```python
from build123d import *

# Parameters (mm, degrees)
SKETCH1_W               = 50.8
SKETCH1_H               = 25.4
SKETCH1_W_2             = 44.45
SKETCH1_H_2             = 19.05
BOSS_EXTRUDE1_DEPTH     = 774.7
SKETCH3_R               = 14.2875
CUT_EXTRUDE2_DEPTH      = 777.578000348
SKETCH2_R               = 6.35
CUT_EXTRUDE1_DEPTH      = 777.578000348
SKETCH4_R               = 2.54
CUT_EXTRUDE3_DEPTH      = 777.578000348
SKETCH5_R               = 2.54
CUT_EXTRUDE4_DEPTH      = 777.578000348
CUT_EXTRUDE5_DEPTH      = 777.578000348
CUT_EXTRUDE5_DEPTH_BACK = 777.578000348
SKETCH6_R               = 3.175
SKETCH8_R               = 2.5796875
CUT_EXTRUDE8_DEPTH      = 777.578000348
SKETCH10_R              = 3.175
SKETCH10_R_2            = 3.3734375
CUT_EXTRUDE9_DEPTH      = 777.578000348
CUT_EXTRUDE10_REACH     = 778.682
SKETCH11_R              = 2.4638
CUT_EXTRUDE11_REACH     = 778.682
SKETCH12_R              = 2.4638
CUT_EXTRUDE12_REACH     = 778.682
SKETCH13_R              = 2.4638


with BuildPart() as part:
    # Sketch1 → Boss-Extrude1 (new body)
    with BuildSketch(Plane(origin=(0, 0, 0), x_dir=(1, 0, 0), z_dir=(0, 1, 0))):
        with Locations((22.225, 9.525)):
            Rectangle(SKETCH1_W, SKETCH1_H)
        with Locations((22.225, 9.525)):
            Rectangle(SKETCH1_W_2, SKETCH1_H_2, mode=Mode.SUBTRACT)
    extrude(amount=BOSS_EXTRUDE1_DEPTH)

    # Sketch3 → Cut-Extrude2 (cut, through all)
    with BuildSketch(Plane.XY.offset(3.175)):
        with Locations((22.225, 81.28)):
            Circle(SKETCH3_R)
    extrude(amount=-CUT_EXTRUDE2_DEPTH, mode=Mode.SUBTRACT)

    # Sketch2 → Cut-Extrude1 (cut, through all)
    with BuildSketch(Plane.XY.offset(3.175)):
        with Locations((22.225, 633.476)):
            Circle(SKETCH2_R)
    extrude(amount=-CUT_EXTRUDE1_DEPTH, mode=Mode.SUBTRACT)

    # Sketch4 → Cut-Extrude3 (cut, through all)
    with BuildSketch(Plane.XY.offset(3.175)):
        with Locations((40.511702836, 42.589037005)):
            Circle(SKETCH4_R)
        with Locations((40.511702836, 119.970962995)):
            Circle(SKETCH4_R)
    extrude(amount=-CUT_EXTRUDE3_DEPTH, mode=Mode.SUBTRACT)

    # Sketch5 → Cut-Extrude4 (cut, through all)
    with BuildSketch(Plane(origin=(0, 0, -22.225), x_dir=(-1, 0, 0), z_dir=(0, 0, -1))):
        with Locations((-10.31875, 612.853770072)):
            Circle(SKETCH5_R)
        with Locations((-34.13125, 612.853770072)):
            Circle(SKETCH5_R)
        with Locations((-10.31875, 654.098229928)):
            Circle(SKETCH5_R)
        with Locations((-34.13125, 654.098229928)):
            Circle(SKETCH5_R)
    extrude(amount=-CUT_EXTRUDE4_DEPTH, mode=Mode.SUBTRACT)

    # Sketch6 → Cut-Extrude5 (cut, two sides: drawn at the far end of the back side and taken through both)
    with BuildSketch(Plane.XY.offset(3.175).offset(-CUT_EXTRUDE5_DEPTH_BACK)):
        with Locations((4.445, 227.076)):
            Circle(SKETCH6_R)
        with Locations((4.445, 328.676)):
            Circle(SKETCH6_R)
    extrude(amount=CUT_EXTRUDE5_DEPTH + CUT_EXTRUDE5_DEPTH_BACK, mode=Mode.SUBTRACT)

    # Sketch8 → Cut-Extrude8 (cut, through all)
    with BuildSketch(Plane.XY.offset(3.175)):
        with Locations((4.445, 315.976)):
            Circle(SKETCH8_R)
        with Locations((4.445, 308.356)):
            Circle(SKETCH8_R)
    extrude(amount=-CUT_EXTRUDE8_DEPTH, mode=Mode.SUBTRACT)

    # Sketch10 → Cut-Extrude9 (cut, through all)
    with BuildSketch(Plane.XY.offset(3.175)):
        with Locations((34.925, 195.58)):
            Circle(SKETCH10_R)
        with Locations((34.925, 391.16)):
            Circle(SKETCH10_R)
        with Locations((34.925, 533.4)):
            Circle(SKETCH10_R)
        with Locations((34.925, 728.98)):
            Circle(SKETCH10_R)
        with Locations((4.445, 728.98)):
            Circle(SKETCH10_R_2)
    extrude(amount=-CUT_EXTRUDE9_DEPTH, mode=Mode.SUBTRACT)

    # Sketch11 → Cut-Extrude10 (cut, up to next)
    with BuildSketch(Plane.ZY.offset(3.175), mode=Mode.PRIVATE) as cut_extrude10_sk1:
        with Locations((-9.525, 762)):
            Circle(SKETCH11_R)
    cut_extrude10_tool1 = extrude(cut_extrude10_sk1.sketch, amount=-CUT_EXTRUDE10_REACH, mode=Mode.PRIVATE) & part.part
    # Sketch11 → Cut-Extrude10 (cut, up to next)
    with BuildSketch(Plane.ZY.offset(3.175), mode=Mode.PRIVATE) as cut_extrude10_sk2:
        with Locations((-9.525, 723.9)):
            Circle(SKETCH11_R)
    cut_extrude10_tool2 = extrude(cut_extrude10_sk2.sketch, amount=-CUT_EXTRUDE10_REACH, mode=Mode.PRIVATE) & part.part
    # Sketch11 → Cut-Extrude10 (cut, up to next)
    with BuildSketch(Plane.ZY.offset(3.175), mode=Mode.PRIVATE) as cut_extrude10_sk3:
        with Locations((-9.525, 558.8)):
            Circle(SKETCH11_R)
    cut_extrude10_tool3 = extrude(cut_extrude10_sk3.sketch, amount=-CUT_EXTRUDE10_REACH, mode=Mode.PRIVATE) & part.part
    # Sketch11 → Cut-Extrude10 (cut, up to next)
    with BuildSketch(Plane.ZY.offset(3.175), mode=Mode.PRIVATE) as cut_extrude10_sk4:
        with Locations((-9.525, 533.4)):
            Circle(SKETCH11_R)
    cut_extrude10_tool4 = extrude(cut_extrude10_sk4.sketch, amount=-CUT_EXTRUDE10_REACH, mode=Mode.PRIVATE) & part.part
    # Sketch11 → Cut-Extrude10 (cut, up to next)
    with BuildSketch(Plane.ZY.offset(3.175), mode=Mode.PRIVATE) as cut_extrude10_sk5:
        with Locations((-9.525, 495.3)):
            Circle(SKETCH11_R)
    cut_extrude10_tool5 = extrude(cut_extrude10_sk5.sketch, amount=-CUT_EXTRUDE10_REACH, mode=Mode.PRIVATE) & part.part
    # Sketch11 → Cut-Extrude10 (cut, up to next)
    with BuildSketch(Plane.ZY.offset(3.175), mode=Mode.PRIVATE) as cut_extrude10_sk6:
        with Locations((-9.525, 50.8)):
            Circle(SKETCH11_R)
    cut_extrude10_tool6 = extrude(cut_extrude10_sk6.sketch, amount=-CUT_EXTRUDE10_REACH, mode=Mode.PRIVATE) & part.part
    # Sketch11 → Cut-Extrude10 (cut, up to next)
    with BuildSketch(Plane.ZY.offset(3.175), mode=Mode.PRIVATE) as cut_extrude10_sk7:
        with Locations((-9.525, 12.7)):
            Circle(SKETCH11_R)
    cut_extrude10_tool7 = extrude(cut_extrude10_sk7.sketch, amount=-CUT_EXTRUDE10_REACH, mode=Mode.PRIVATE) & part.part
    add(cut_extrude10_tool1.solids().sort_by_distance((-3.175, 762, -9.525))[0], mode=Mode.SUBTRACT)
    add(cut_extrude10_tool2.solids().sort_by_distance((-3.175, 723.9, -9.525))[0], mode=Mode.SUBTRACT)
    add(cut_extrude10_tool3.solids().sort_by_distance((-3.175, 558.8, -9.525))[0], mode=Mode.SUBTRACT)
    add(cut_extrude10_tool4.solids().sort_by_distance((-3.175, 533.4, -9.525))[0], mode=Mode.SUBTRACT)
    add(cut_extrude10_tool5.solids().sort_by_distance((-3.175, 495.3, -9.525))[0], mode=Mode.SUBTRACT)
    add(cut_extrude10_tool6.solids().sort_by_distance((-3.175, 50.8, -9.525))[0], mode=Mode.SUBTRACT)
    add(cut_extrude10_tool7.solids().sort_by_distance((-3.175, 12.7, -9.525))[0], mode=Mode.SUBTRACT)

    # Sketch12 → Cut-Extrude11 (cut, up to next)
    with BuildSketch(Plane(origin=(47.625, 0, 0), x_dir=(0, 0, -1), z_dir=(1, 0, 0)), mode=Mode.PRIVATE) as cut_extrude11_sk1:
        with Locations(Location((9.525, 50.8, 0), (0, 0, 180))):
            Circle(SKETCH12_R)
    cut_extrude11_tool1 = extrude(cut_extrude11_sk1.sketch, amount=-CUT_EXTRUDE11_REACH, mode=Mode.PRIVATE) & part.part
    # Sketch12 → Cut-Extrude11 (cut, up to next)
    with BuildSketch(Plane(origin=(47.625, 0, 0), x_dir=(0, 0, -1), z_dir=(1, 0, 0)), mode=Mode.PRIVATE) as cut_extrude11_sk2:
        with Locations((9.525, 114.3)):
            Circle(SKETCH12_R)
    cut_extrude11_tool2 = extrude(cut_extrude11_sk2.sketch, amount=-CUT_EXTRUDE11_REACH, mode=Mode.PRIVATE) & part.part
    # Sketch12 → Cut-Extrude11 (cut, up to next)
    with BuildSketch(Plane(origin=(47.625, 0, 0), x_dir=(0, 0, -1), z_dir=(1, 0, 0)), mode=Mode.PRIVATE) as cut_extrude11_sk3:
        with Locations((9.525, 177.8)):
            Circle(SKETCH12_R)
    cut_extrude11_tool3 = extrude(cut_extrude11_sk3.sketch, amount=-CUT_EXTRUDE11_REACH, mode=Mode.PRIVATE) & part.part
    # Sketch12 → Cut-Extrude11 (cut, up to next)
    with BuildSketch(Plane(origin=(47.625, 0, 0), x_dir=(0, 0, -1), z_dir=(1, 0, 0)), mode=Mode.PRIVATE) as cut_extrude11_sk4:
        with Locations((9.525, 241.3)):
            Circle(SKETCH12_R)
    cut_extrude11_tool4 = extrude(cut_extrude11_sk4.sketch, amount=-CUT_EXTRUDE11_REACH, mode=Mode.PRIVATE) & part.part
    # Sketch12 → Cut-Extrude11 (cut, up to next)
    with BuildSketch(Plane(origin=(47.625, 0, 0), x_dir=(0, 0, -1), z_dir=(1, 0, 0)), mode=Mode.PRIVATE) as cut_extrude11_sk5:
        with Locations((9.525, 304.8)):
            Circle(SKETCH12_R)
    cut_extrude11_tool5 = extrude(cut_extrude11_sk5.sketch, amount=-CUT_EXTRUDE11_REACH, mode=Mode.PRIVATE) & part.part
    # Sketch12 → Cut-Extrude11 (cut, up to next)
    with BuildSketch(Plane(origin=(47.625, 0, 0), x_dir=(0, 0, -1), z_dir=(1, 0, 0)), mode=Mode.PRIVATE) as cut_extrude11_sk6:
        with Locations((9.525, 368.3)):
            Circle(SKETCH12_R)
    cut_extrude11_tool6 = extrude(cut_extrude11_sk6.sketch, amount=-CUT_EXTRUDE11_REACH, mode=Mode.PRIVATE) & part.part
    # Sketch12 → Cut-Extrude11 (cut, up to next)
    with BuildSketch(Plane(origin=(47.625, 0, 0), x_dir=(0, 0, -1), z_dir=(1, 0, 0)), mode=Mode.PRIVATE) as cut_extrude11_sk7:
        with Locations((9.525, 431.8)):
            Circle(SKETCH12_R)
    cut_extrude11_tool7 = extrude(cut_extrude11_sk7.sketch, amount=-CUT_EXTRUDE11_REACH, mode=Mode.PRIVATE) & part.part
    # Sketch12 → Cut-Extrude11 (cut, up to next)
    with BuildSketch(Plane(origin=(47.625, 0, 0), x_dir=(0, 0, -1), z_dir=(1, 0, 0)), mode=Mode.PRIVATE) as cut_extrude11_sk8:
        with Locations(Location((9.525, 495.3, 0), (0, 0, 180))):
            Circle(SKETCH12_R)
    cut_extrude11_tool8 = extrude(cut_extrude11_sk8.sketch, amount=-CUT_EXTRUDE11_REACH, mode=Mode.PRIVATE) & part.part
    # Sketch12 → Cut-Extrude11 (cut, up to next)
    with BuildSketch(Plane(origin=(47.625, 0, 0), x_dir=(0, 0, -1), z_dir=(1, 0, 0)), mode=Mode.PRIVATE) as cut_extrude11_sk9:
        with Locations(Location((9.525, 558.8, 0), (0, 0, 180))):
            Circle(SKETCH12_R)
    cut_extrude11_tool9 = extrude(cut_extrude11_sk9.sketch, amount=-CUT_EXTRUDE11_REACH, mode=Mode.PRIVATE) & part.part
    add(cut_extrude11_tool1.solids().sort_by_distance((47.625, 50.8, -9.525))[0], mode=Mode.SUBTRACT)
    add(cut_extrude11_tool2.solids().sort_by_distance((47.625, 114.3, -9.525))[0], mode=Mode.SUBTRACT)
    add(cut_extrude11_tool3.solids().sort_by_distance((47.625, 177.8, -9.525))[0], mode=Mode.SUBTRACT)
    add(cut_extrude11_tool4.solids().sort_by_distance((47.625, 241.3, -9.525))[0], mode=Mode.SUBTRACT)
    add(cut_extrude11_tool5.solids().sort_by_distance((47.625, 304.8, -9.525))[0], mode=Mode.SUBTRACT)
    add(cut_extrude11_tool6.solids().sort_by_distance((47.625, 368.3, -9.525))[0], mode=Mode.SUBTRACT)
    add(cut_extrude11_tool7.solids().sort_by_distance((47.625, 431.8, -9.525))[0], mode=Mode.SUBTRACT)
    add(cut_extrude11_tool8.solids().sort_by_distance((47.625, 495.3, -9.525))[0], mode=Mode.SUBTRACT)
    add(cut_extrude11_tool9.solids().sort_by_distance((47.625, 558.8, -9.525))[0], mode=Mode.SUBTRACT)

    # Sketch13 → Cut-Extrude12 (cut, up to next)
    with BuildSketch(Plane(origin=(47.625, 0, 0), x_dir=(0, 0, -1), z_dir=(1, 0, 0)), mode=Mode.PRIVATE) as cut_extrude12_sk1:
        with Locations(Location((9.525, 762, 0), (0, 0, 180))):
            Circle(SKETCH13_R)
    cut_extrude12_tool1 = extrude(cut_extrude12_sk1.sketch, amount=-CUT_EXTRUDE12_REACH, mode=Mode.PRIVATE) & part.part
    # Sketch13 → Cut-Extrude12 (cut, up to next)
    with BuildSketch(Plane(origin=(47.625, 0, 0), x_dir=(0, 0, -1), z_dir=(1, 0, 0)), mode=Mode.PRIVATE) as cut_extrude12_sk2:
        with Locations(Location((9.525, 723.9, 0), (0, 0, 180))):
            Circle(SKETCH13_R)
    cut_extrude12_tool2 = extrude(cut_extrude12_sk2.sketch, amount=-CUT_EXTRUDE12_REACH, mode=Mode.PRIVATE) & part.part
    add(cut_extrude12_tool1.solids().sort_by_distance((47.625, 762, -9.525))[0], mode=Mode.SUBTRACT)
    add(cut_extrude12_tool2.solids().sort_by_distance((47.625, 723.9, -9.525))[0], mode=Mode.SUBTRACT)


solid = part.part
```
CAD build for the part. Positions are in the model's coordinates, mm. A direction names the side the tool comes from. Round coordinates to 2 decimals unless told otherwise and drop trailing zeros. Write each loop counter-clockwise with the first axis right and the second up, starting at its lowest first coordinate (ties: lowest second). Pieces come first, ordered by that corner, then holes. Notation, with made-up numbers: (41.25, 34.5) - (96.25, 34.5) arc R21 cw to (96.25, 64.5) - close; hole circle Ø4 at (27.25, 35.25). An arc over 180 degrees is marked (long way). Return JSON: item names as keys, results as strings. Group by question number.
Item 1: 3-axis set-ups, long thin cutter, end or side, ignore diameter. For faces 4 (the face through (-3.175, 382, -9)), 5 (the face through (22, 382, -19.05)): which of +Z, -Z, +X, -X, +Y, -Y reach the whole face in a straight line?
Item 2: Band-saw the part on B-B on y = 475.5. List the corners of the cut face in (x, z) (3 decimals).
Item 3: Probe probe 1 along Z at (x, y) = (26, 384) (3 decimals); probe 2 along Z at (x, y) = (-2, 762) (3 decimals); probe 3 along X at (y, z) = (150.5, -17.5) (3 decimals). List the from-to ranges inside material, lowest first.
Item 4: Mould opens along Y. For faces 1 (the face through (0, 382, -9)), 2 (the face through (25.64, 638.83, 1.61)), 3 (the face through (22, 0, -20)) say: +Y half, -Y half, draft (parallel to the pull), parting line (faces both ways), or undercut.
Resolved:
{
 "1": {"face 4": "+Z, -Z, -X, +Y, -Y", "face 5": "+Y, -Y"},
 "2": {"outline": "(-3.175, -22.225) - (47.625, -22.225) - (47.625, 3.175) - (-3.175, 3.175) - close; hole (0, -19.05) - (44.45, -19.05) - (44.45, 0) - (0, 0) - close"},
 "3": {"probe 1": "z = -22.225 to -19.05, 0 to 3.175", "probe 2": "z = -22.225 to -11.989, -7.061 to 3.175", "probe 3": "x = -3.175 to 0, 44.45 to 47.625"},
 "4": {"face 1": "draft", "face 2": "undercut", "face 3": "-Y half"}
}
